```python
from build123d import *

# Parameters (mm, degrees)
EXTRUDE_1_DEPTH      = 20
EXTRUDE_1_DEPTH_BACK = 42
SKETCH_2_R           = 7.5
CUT_EXTRUDE_1_DEPTH  = 65
EXTRUDE_2_DEPTH      = 5
SKETCH_4_R           = 3
EXTRUDE_3_DEPTH      = 16
SKETCH_5_R           = 9
EXTRUDE_4_DEPTH      = 7
EXTRUDE_5_DEPTH      = 7


with BuildPart() as part:
    # 草图1 → 凸台-拉伸1 (new body, two sides)
    with BuildSketch(Plane.XY) as extrude_1_sk:
        Polygon((-6.639528096, -11.5), (6.639528096, -11.5), (13.279056191, 0), (6.639528096, 11.5), (-6.639528096, 11.5), (-13.279056191, 0), align=None)
    extrude(amount=EXTRUDE_1_DEPTH)
    extrude(extrude_1_sk.sketch, amount=-EXTRUDE_1_DEPTH_BACK)

    # 草图2 → 切除-拉伸1 (cut)
    with BuildSketch(Plane.XY.offset(20)):
        Circle(SKETCH_2_R)
    extrude(amount=-CUT_EXTRUDE_1_DEPTH, mode=Mode.SUBTRACT)

    # 草图3 → 凸台-拉伸2 (add)
    with BuildSketch(Plane(origin=(9.959292144, 5.75, 0), x_dir=(0, 0, -1), z_dir=(0.866025404, 0.5, 0))):
        Polygon((-3.020588915, -5.357215685), (3.041588911, -5.357215685), (6.072677825, -0.107215685), (3.041588911, 5.142784315), (-3.020588915, 5.142784315), (-6.051677828, -0.107215685), align=None)
    extrude(amount=EXTRUDE_2_DEPTH)

    # 草图4 → 凸台-拉伸3 (add)
    with BuildSketch(Plane(origin=(14.289419162, 8.25, 0), x_dir=(0, 0, -1), z_dir=(0.866025404, 0.5, 0))):
        Circle(SKETCH_4_R)
    extrude(amount=EXTRUDE_3_DEPTH)

    # 草图5 → 凸台-拉伸4 (add)
    with BuildSketch(Plane(origin=(28.145825623, 16.25, 0), x_dir=(0, 0, -1), z_dir=(0.866025404, 0.5, 0))):
        Circle(SKETCH_5_R)
    extrude(amount=EXTRUDE_4_DEPTH)

    # 草图6 → 凸台-拉伸5 (add)
    with BuildSketch(Plane(origin=(-9.959292144, -5.75, 0), x_dir=(0, 0, 1), z_dir=(-0.866025404, -0.5, 0))):
        Polygon((-16.732210102, -5.46), (-10.427545163, -5.46), (-7.275212693, 0), (-10.427545163, 5.46), (-16.732210102, 5.46), (-19.884542572, 0), align=None)
    extrude(amount=EXTRUDE_5_DEPTH)


solid = part.part
```
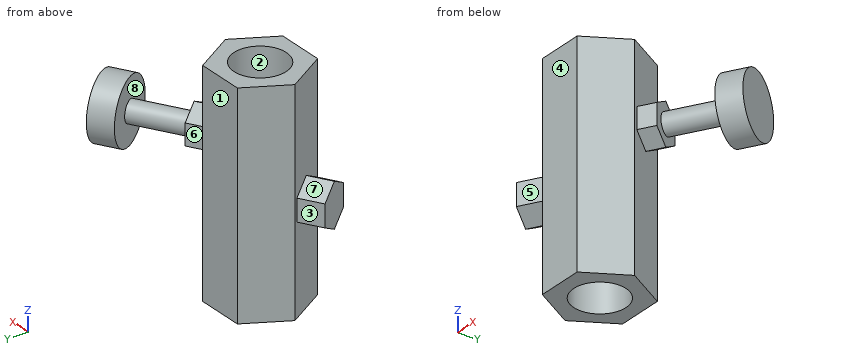
The listing builds one solid part. Answer for the finished solid, in the listing's coordinates (mm). Face numbers are marked on the shaded views. A direction names the side the tool comes from. Coordinates: 2 decimals unless noted, no trailing zeros. Loops run counter-clockwise (first coordinate to the right, second up) from the corner with the lowest first, then second, coordinate; pieces in that order, holes last. Notation, with made-up numbers: M 26.5,12 L 76.5,12 A17 cw 76.5,36 Z; hole C 6.25,11 d2. An arc over 180 degrees is marked long. Answer as a JSON object with one key per item and string values. Group by question number.
Item 1: Section C-C (z = -18.5) is taken. Write down the section's boundary in (x, y), and give its area (3 significant figures).
Item 2: Section A-A (z = 16) is taken. Write down the section's boundary in (x, y), and give its area (3 significant figures).
Item 3: Determine the mould class of the marked faces 1, 2 and 3 for opening direction X: +X half, -X half, draft (parallel to the pull), parting line (faces both ways), or undercut.
Item 4: Which of the six approach directions +Z, -Z, +X, -X, +Y, -Y give full straight-line access (tool end or side, diameter ignored) to the marked faces 4, 5, 6, 7 and 8?
Item 5: Each of these flat-tipped pins is pushed along its axis until it touches: P1, Ø3, axis at x = -11.5, y = 3.5, coming from the -Z side; P2, Ø5, axis at y = 9, z = -10, coming from the -X side; P3, Ø1, axis at y = 11, z = 5, coming from the +X side; P4, Ø4, axis at x = 14.5, z = -20.5, coming from the -Y side. Where does it stop, or does it pass through?
Item 6: Consider L1, parallel to Y at x = 0, z = -19; L2, parallel to X at y = 1.5, z = -9; L3, parallel to Y at x = -3, z = -33. Determine where each line is inside the solid, lowest interval first.
Item 7: Section B-B (x = 0) is taken. Write down the section's boundary in (y, z).
Item 8: Section D-D (x = -9) is taken. Write down the section's boundary in (y, z), and give its area (3 significant figures).
Solved:
{
 "1": {"outline": "M -17.22,-7.17 L -14.82,-11.33 L -8.76,-7.83 L -6.64,-11.5 L 6.64,-11.5 L 13.28,0 L 6.64,11.5 L -6.64,11.5 L -13.28,0 L -11.16,-3.67 Z; hole C 0,0 d15", "area": "315 mm2"},
 "2": {"outline": "M -13.28,0 L -6.64,-11.5 L 6.64,-11.5 L 13.28,0 L 6.64,11.5 L -6.64,11.5 Z; hole C 0,0 d15", "area": "281 mm2"},
 "3": {"face 1": "draft", "face 2": "undercut", "face 3": "-X half"},
 "4": {"face 4": "+Z, -Z, +X, -Y", "face 5": "+Z, -Z, -Y", "face 6": "+Z, -Z, +Y", "face 7": "+Z, -X", "face 8": "none"},
 "5": {"P1": "stops at z = -42", "P2": "stops at x = -9.53", "P3": "stops at x = 35.1", "P4": "stops at y = -1.35"},
 "6": {"L1": "y = -11.5 to -7.5, 7.5 to 11.5", "L2": "x = -12.41 to -7.35, 7.35 to 12.41", "L3": "y = -11.5 to -6.87, 6.87 to 11.5"},
 "7": {"outline": "M -11.5,-42 L -7.5,-42 L -7.5,20 L -11.5,20 Z; M 7.5,-42 L 11.5,-42 L 11.5,20 L 7.5,20 Z"},
 "8": {"outline": "M -11.5,-16.73 L -7.41,-18.78 L -7.41,-42 L 7.41,-42 L 7.41,20 L -7.41,20 L -7.41,-8.38 L -11.5,-10.43 Z", "area": "953 mm2"}
}
